from build123d import *

# Parameters (mm, degrees)
BOSS_EXTRUDE1_DEPTH     = 5
SKETCH3_R               = 1.25
CUT_EXTRUDE1_DEPTH      = 300
CUT_EXTRUDE1_DEPTH_BACK = 11
SKETCH4_R               = 1
CUT_EXTRUDE2_DEPTH      = 11


with BuildPart() as part:
    # Sketch2 → Boss-Extrude1 (new body)
    with BuildSketch(Plane.XY):
        with BuildLine():
            ThreePointArc((-8, 0), (0, 8), (8, 0))
            Line((8, 0), (13.6, 0))
            Line((13.6, 0), (13.6, 10))
            Line((13.6, 10), (8.008871246, 10))
            ThreePointArc((8.008871246, 10), (6.357463889, 8.822466805), (4.337930538, 9.01012534))
            ThreePointArc((4.337930538, 9.01012534), (0.001186479, 9.99999993), (-4.335792351, 9.011154459))
            ThreePointArc((-4.335792351, 9.011154459), (-6.353531515, 8.82385013), (-8.003690819, 10))
            Line((-8.003690819, 10), (-13.6, 10))
            Line((-13.6, 10), (-13.6, 0))
            Line((-13.6, 0), (-8, 0))
        make_face()
    extrude(amount=BOSS_EXTRUDE1_DEPTH)

    # Sketch3 → Cut-Extrude1 (cut, two sides)
    with BuildSketch(Plane(origin=(0, 10, 0), x_dir=(1, 0, 0), z_dir=(0, 1, 0))) as cut_extrude1_sk:
        with Locations((-10.998930891, -2.5)):
            Circle(SKETCH3_R)
        with Locations((11.001069109, -2.5)):
            Circle(SKETCH3_R)
    extrude(amount=CUT_EXTRUDE1_DEPTH, mode=Mode.SUBTRACT)
    extrude(cut_extrude1_sk.sketch, amount=-CUT_EXTRUDE1_DEPTH_BACK, mode=Mode.SUBTRACT)

    # Sketch4 → Cut-Extrude2 (cut, through all)
    with BuildSketch(Plane(origin=(0, 10, 0), x_dir=(1, 0, 0), z_dir=(0, 1, 0))):
        with Locations((0, -2.5)):
            Circle(SKETCH4_R)
    extrude(amount=-CUT_EXTRUDE2_DEPTH, mode=Mode.SUBTRACT)


solid = part.part
Check sheet for the modelled part. Datum: model origin and axes. Units: mm. Round coordinates to 2 decimals unless told otherwise and drop trailing zeros. Order: outer loops, then holes, each group sorted by start corner. A loop starts at its lowest first (then second) coordinate and runs counter-clockwise, first axis right, second up.
(1) Cross-section at C-C, the plane z = 2.2. Enter the section's corners in (x, y), and give its area (3 significant figures).
(2) Draft check along Z on faces 1 (the cylindrical face through (-10.327, 5.07, 1.446)), 2 (the cylindrical face through (-0.217, 8.982, 3.476)), 3 (the flat face through (-9.59, 0, 2.46)), 4 (the flat face through (-0.2, 8.4, 0)). Enter one of: pulls with the +Z half, pulls with the -Z half, needs draft (parallel to the pull), parting line crosses it, or undercut.
(3) Cross-section at A-A, the plane x = 0. Enter the section's corners in (y, z), and give its area (3 significant figures).
(4) Cross-section at D-D, the plane y = 1. Enter the section's corners in (x, z).
(5) Scan lines: probe 1 along Z at (x, y) = (0, 9.3); probe 2 along X at (y, z) = (5.25, 2.5); probe 3 along X at (y, z) = (5.25, 2.15). Record each from-to range of solid material in increasing order.
(6) Cross-section at B-B, the plane y = 7.5. Enter the section's corners in (x, z).
(7) Go/stop test with flat-tipped pins: P1, Ø1.5, axis at x = 6.5, y = 9, coming from the -Z side; P2, Ø1.5, axis at x = 1.5, z = 3.5, coming from the +Y side; P3, Ø2, axis at x = 11, z = 2.5, coming from the +Y side; P4, Ø3, axis at x = 3, z = 1, coming from the +Y side. Record where each tip stops, or that it passes through.
Check sheet entries:
1. outline: (-13.6, 0) - (-12.21, 0) - (-12.21, 10) - (-13.6, 10) - close; (-9.79, 0) - (-8, 0) arc R8 cw to (-0.95, 7.94) - (-0.95, 9.95) arc R10 ccw to (-4.34, 9.01) arc R2.91 cw to (-8, 10) - (-9.79, 10) - close; (0.95, 7.94) arc R8 cw to (8, 0) - (9.79, 0) - (9.79, 10) - (8.01, 10) arc R2.91 cw to (4.34, 9.01) arc R10 ccw to (0.95, 9.95) - close; (12.21, 0) - (13.6, 0) - (13.6, 10) - (12.21, 10) - close
1. area: 109 mm2
2. face 1: undercut
2. face 2: undercut
2. face 3: needs draft
2. face 4: pulls with the -Z half
3. outline: (8, 0) - (10, 0) - (10, 1.5) - (8, 1.5) - close; (8, 3.5) - (10, 3.5) - (10, 5) - (8, 5) - close
3. area: 6.00 mm2
4. outline: (-13.6, 0) - (-7.94, 0) - (-7.94, 5) - (-13.6, 5) - close; (7.94, 0) - (13.6, 0) - (13.6, 5) - (7.94, 5) - close; hole circle Ø2.5 at (-11, 2.5); hole circle Ø2.5 at (11, 2.5)
5. probe 1: z = 0 to 1.5, 3.5 to 5
5. probe 2: x = -13.6 to -12.25, -9.75 to -6.04, 6.04 to 9.75, 12.25 to 13.6
5. probe 3: x = -13.6 to -12.2, -9.8 to -6.04, 6.04 to 9.8, 12.2 to 13.6
6. outline: (-13.6, 0) - (-2.78, 0) - (-2.78, 5) - (-13.6, 5) - close; (2.78, 0) - (13.6, 0) - (13.6, 5) - (2.78, 5) - close; hole circle Ø2.5 at (-11, 2.5); hole circle Ø2.5 at (11, 2.5)
7. P1: stops at z = 0
7. P2: stops at y = 9.97
7. P3: passes through
7. P4: stops at y = 9.89
